```python
from build123d import *

# Parameters (mm, degrees)
F0_R     = 3.175
F1_DEPTH = 127
F2_R     = 2.032
F3_DEPTH = 6.35
F5_DEPTH = 12.7


with BuildPart() as f1:
    # F0 (on Front) → F1 (new body)
    with BuildSketch(Plane.XZ):
        Circle(F0_R)
    extrude(amount=F1_DEPTH)

    # F2 (on Right) → F3 (join)
    with BuildSketch(Plane.YZ):
        with Locations((-123.687468, 0)):
            Circle(F2_R)
    extrude(amount=-F3_DEPTH)

    # F4 (on Right) → F5 (cut, symmetric)
    with BuildSketch(Plane.YZ):
        Polygon((0.1524, -3.522164), (0.1524, 3.558817), (-6.928581, 3.558817), align=None)
    extrude(amount=F5_DEPTH, both=True, mode=Mode.SUBTRACT)


solid = f1.part
```
The model under review builds one solid part; all positions refer to its coordinate system, in mm. A direction names the side the tool comes from. Round coordinates to 2 decimals unless told otherwise and drop trailing zeros. Order: outer loops, then holes, each group sorted by start corner. A loop starts at its lowest first (then second) coordinate and runs counter-clockwise, first axis right, second up. Notation, with made-up numbers: (73, 59.25) -> (108, 59.25) arc R9 cw to (108, 65.25) -> close; hole circle Ø11 at (9, -19.5). An arc over 180 degrees is marked (long way). Use a Markdown table: item, result.
Q1. We need section B-B on x = 0. Write out the cut boundary in (y, z) (3 decimals), then the cut area to 3 significant figures.
Values:
| item | result |
|---|---|
| outline | (-127, -3.175) -> (-0.195, -3.175) -> (-6.545, 3.175) -> (-127, 3.175) -> close |
| area | 785 mm^2 |
Q2. We need section C-C on y = -75.5. Write out the cut boundary in (x, z) (3 decimals).
Values:
| item | result |
|---|---|
| outline | circle Ø6.35 at (0, 0) |
Q3. Tool access review of faces 1 (the flat face through (0, -127, 0)), 2 (the cylindrical face through (-4.367, -125.3, -1.236)): name each direction out of +Z, -Z, +X, -X, +Y, -Y from which nothing blocks a thin tool from reaching the whole face with its end or side.
Values:
| item | result |
|---|---|
| face 1 | +Z, -Z, +X, -X, -Y |
| face 2 | -X |
Q4. For line 1 (X direction, y = -47, z = 0) (3 decimals); line 2 (Z direction, x = 0.25, y = -48); line 3 (Y direction, x = -4, z = -0.25), list the stretches that pass through material, from the lowest coordinate up.
Values:
| item | result |
|---|---|
| line 1 | x = -3.175 to 3.175 |
| line 2 | z = -3.17 to 3.17 |
| line 3 | y = -125.7 to -121.67 |
Q5. Clearance check with a flat-ended pin moving along its axis: P1, Ø2, axis at y = -57, z = -2.5, coming from the +X side. State where the tip first meets the part, or that it passes through.
Values:
| item | result |
|---|---|
| P1 | stops at x = 2.8 |
Q6. We need section A-A on z = 0. Write out the cut boundary in (x, y) (3 decimals), then the cut area to 3 significant figures.
Values:
| item | result |
|---|---|
| outline | (-6.35, -125.719) -> (-3.175, -125.719) -> (-3.175, -127) -> (3.175, -127) -> (3.175, -3.37) -> (-3.175, -3.37) -> (-3.175, -121.655) -> (-6.35, -121.655) -> close |
| area | 798 mm^2 |
